Check sheet for the modelled part. Datum: model origin and axes. Units: mm. Give positions to 0.01 mm unless a question says otherwise; leave off trailing zeros. Loops run counter-clockwise (first coordinate to the right, second up) from the corner with the lowest first, then second, coordinate; pieces in that order, holes last. Notation, with made-up numbers: M 1,25 L 43,25 A25 cw 43,46 Z; hole C -13,32.5 d6. An arc over 180 degrees is marked long. Put each result on its own line as item: value. Start each with the question number.
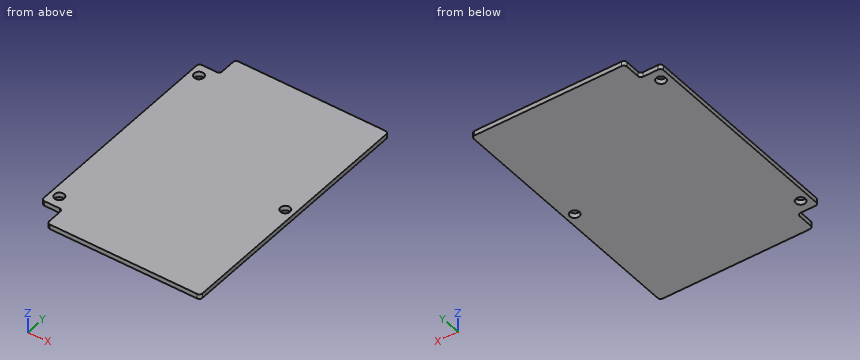
Autodesk Inventor part; units mm, degrees
ref_plane "YZ Plane" through (0, 0, 0) normal (1, 0, 0) x (0, 1, 0)
ref_plane "XZ Plane" through (0, 0, 0) normal (0, 1, 0) x (-1, 0, 0)
ref_plane "XY Plane" through (0, 0, 0) normal (0, 0, 1) x (1, 0, 0)
sketch "Skizze1" plane through (0, 0, 0) normal (0, 0, 1) x (1, 0, 0)
  line L0 (-22, -42.5) -> (29, -42.5)
  line L1 (29, -42.5) -> (29, 42.5)
  line L2 (29, 42.5) -> (-22, 42.5)
  line L3 (-29, 35.5) -> (-29, -35.5)
  line L4 (-22, -42.5) -> (-22, -35.5)
  line L5 (-22, -35.5) -> (-29, -35.5)
  line L6 (-22, 42.5) -> (-22, 35.5)
  line L7 (-22, 35.5) -> (-29, 35.5)
  line L8 (0, 59.5) -> (0, -59.5)
  line L9 (-40.6, 0) -> (40.6, 0)
  dimension "d22" = 58
  dimension "d23" = 85
  dimension "d24" = 7
  dimension "d25" = 7
  dimension "d26" = 7
  dimension "d27" = 7
extrude "Extrusion1" add sketch "Skizze1" along normal blind 1.6
sketch "Skizze2" plane through (0, 0, 1.6) normal (0, 0, 1) x (1, 0, 0)
  line L0 (-22, -42.5) -> (29, -42.5)
  line L1 (29, -42.5) -> (29, 42.5)
  line L2 (29, 42.5) -> (-22, 42.5)
  line L3 (-29, 35.5) -> (-29, -35.5)
  line L4 (-22, 42.5) -> (-22, 35.5)
  line L5 (-22, 35.5) -> (-29, 35.5)
  line L6 (-29, -35.5) -> (-22, -35.5)
  line L7 (-22, -35.5) -> (-22, -42.5)
  line L8 (-40.6, 0) -> (40.6, 0)
  point P0 (0, 0)
  point P1 (-26, 31.5)
  point P2 (-26, -31.5)
  point P3 (26, 0)
  dimension "d28" = 55
  dimension "d29" = 11
  dimension "d30" = 3
  dimension "d31" = 3
  dimension "d32" = 11
hole "Bohrung1" at (-26, 31.5, 1.6) at (-26, -31.5, 1.6) at (26, 0, 1.6) direction (0, 0, -1) diameter 3.2 end through all
fillet "Rundung1" radius 1 8 edges at (29, -42.5, 0.8) (29, 42.5, 0.8) (-22, -35.5, 0.8) (-22, -42.5, 0.8) (-29, -35.5, 0.8) (-29, 35.5, 0.8) (-22, 35.5, 0.8) (-22, 42.5, 0.8)
equation "\"d26\" = d24"
equation "\"d27\" = d25"
properties part number "Base Station PCB" material "Phenolharz"
Q1. Section check B-B, the plane y = 0. Record the cut outline in (x, z), then the cut area to 3 significant figures.
Q2. Thickness scan on line 1 along X through (y, z) = (-31.5, 0.85); line 2 along Y through (x, z) = (-25.5, 0.7); line 3 along Y through (x, z) = (26, 0.55). Record the ranges inside material, lowest first. Write a range as [from, to].
Q3. Section check C-C, the plane z = 0.7. Record the cut outline in (x, y), then the cut area to 3 significant figures.
Q4. Section check A-A, the plane x = -26. Record the cut outline in (y, z), then the cut area to 3 significant figures.
Q5. Depth check by flat-ended pin: P1, Ø3.5, axis at x = -26, y = 31.5, coming from the +Z side; P2, Ø0.5, axis at x = -25, z = 1, coming from the -Y side; P3, Ø0.5, axis at x = -25, z = 0.5, coming from the +Y side; P4, Ø0.5, axis at y = -39, z = 0.5, coming from the -X side. Enter the tip coordinate at first touch or a pass-through.
Found:
1. outline: M -29,0 L 24.4,0 L 24.4,1.6 L -29,1.6 Z; M 27.6,0 L 29,0 L 29,1.6 L 27.6,1.6 Z
1. area: 87.7 mm^2
2. line 1: x = [-29, -27.6], [-24.4, 29]
2. line 2: y = [-35.5, -33.02], [-29.98, 29.98], [33.02, 35.5]
2. line 3: y = [-42.5, -1.6], [1.6, 42.5]
3. outline: M -29,-34.5 A1 ccw -28,-35.5 L -23,-35.5 A1 cw -22,-36.5 L -22,-41.5 A1 ccw -21,-42.5 L 28,-42.5 A1 ccw 29,-41.5 L 29,41.5 A1 ccw 28,42.5 L -21,42.5 A1 ccw -22,41.5 L -22,36.5 A1 cw -23,35.5 L -28,35.5 A1 ccw -29,34.5 Z; hole C -26,-31.5 d3.2; hole C -26,31.5 d3.2; hole C 26,0 d3.2
3. area: 4,810 mm^2
4. outline: M -35.5,0 L -33.1,0 L -33.1,1.6 L -35.5,1.6 Z; M -29.9,0 L 29.9,0 L 29.9,1.6 L -29.9,1.6 Z; M 33.1,0 L 35.5,0 L 35.5,1.6 L 33.1,1.6 Z
4. area: 103 mm^2
5. P1: stops at z = 1.6
5. P2: stops at y = -35.5
5. P3: stops at y = 35.5
5. P4: stops at x = -22
